Can you work these out from the model? Positions are in its coordinate system, mm. Round coordinates to 2 decimals unless told otherwise and drop trailing zeros. Write each loop counter-clockwise with the first axis right and the second up, starting at its lowest first coordinate (ties: lowest second). Pieces come first, ordered by that corner, then holes. Notation, with made-up numbers: (-31.5, 32) - (16.5, 32) arc R19 ccw to (16.5, 49) - close; hole circle Ø4 at (59, 37.5). An arc over 180 degrees is marked (long way). One line per item, written item: value. Start each with the question number.
(1) If I drill on L1, parallel to X at y = 3.5, z = 0.25; L2, parallel to Z at x = -36, y = 0.25; L3, parallel to X at y = 3.25, z = 1.5, over which ranges is the centre line in solid material (lowest first)? Write a range as from..to.
(2) I want a section at C-C on x = 1.5. List the corners of the cut face in (y, z) for me, plus the area to 3 significant figures.
(3) I want a section at B-B on y = 5.5. Give the number of separate pieces and of enclosed holes in the cut face, plus the area to 3 significant figures.
(4) I want a section at A-A on z = 0. List the corners of the cut face in (x, y) for me, plus the area to 3 significant figures.
(5) I want a section at D-D on x = 36. List the corners of the cut face in (y, z) for me, plus the area to 3 significant figures.
(6) I'm going to push flat-ended pins straight in: pin 1 Ø2 at (x, z) = (-2.5, 3.5) entering from +Y; pin 2 Ø1 at (x, y) = (-9, 1) entering from -Z; pin 3 Ø2 at (x, z) = (13, -2.5) entering from +Y. Where does each tip first touch, or does it pass through?
from build123d import *

# Parameters (mm, degrees)
DODANIE_WYCI_GNI_CIE1_DEPTH                 = 41
DODANIE_WYCI_GNI_CIE1_DEPTH_BACK            = 41
SZKIC2_R                                    = 7.5
WYTNIJ_WYCI_GNI_CIE1_REACH                  = 44.35
WYTNIJ_WYCI_GNI_CIE1_END_RADIUS             = 7.5
SZKIC3_R                                    = 2.5
WYTNIJ_WYCI_GNI_CIE1_DIRECTION_2_REACH      = 44.35
WYTNIJ_WYCI_GNI_CIE1_DIRECTION_2_END_RADIUS = 7.5
SFAZOWANIE1_SIZE                            = 1


with BuildPart() as part:
    # Szkic2 → Dodanie-wyciągnięcie1 (new, two sides: drawn at the far end of the back side and taken through both)
    with BuildSketch(Plane(origin=(0, 0, 0), x_dir=(0, 0, -1), z_dir=(1, 0, 0)).offset(-DODANIE_WYCI_GNI_CIE1_DEPTH_BACK)):
        Circle(SZKIC2_R)
    extrude(amount=DODANIE_WYCI_GNI_CIE1_DEPTH + DODANIE_WYCI_GNI_CIE1_DEPTH_BACK)

    # Wytnij-wyciągnięcie1: up to this cylinder (the profile starts inside it)
    wytnij_wyci_gni_cie1_end = Plane(origin=(0, 0, 0), z_dir=(1, 0, 0)) * Cylinder(WYTNIJ_WYCI_GNI_CIE1_END_RADIUS, 176.7, mode=Mode.PRIVATE)
    # Szkic3 → Wytnij-wyciągnięcie1 (cut, up to the surface)
    with BuildSketch(Plane(origin=(0, 0, 0), x_dir=(1, 0, 0), z_dir=(0, 1, 0)), mode=Mode.PRIVATE) as wytnij_wyci_gni_cie1_sk1:
        with Locations(Location((-36, 0, 0), (0, 0, 90))):
            Circle(SZKIC3_R)
    wytnij_wyci_gni_cie1_tool1 = extrude(wytnij_wyci_gni_cie1_sk1.sketch, amount=-WYTNIJ_WYCI_GNI_CIE1_REACH, mode=Mode.PRIVATE) & wytnij_wyci_gni_cie1_end
    add(wytnij_wyci_gni_cie1_tool1.solids().sort_by_distance((-36, 0, 0))[0], mode=Mode.SUBTRACT)
    # Szkic3 → Wytnij-wyciągnięcie1 (cut, up to the surface)
    with BuildSketch(Plane(origin=(0, 0, 0), x_dir=(1, 0, 0), z_dir=(0, 1, 0)), mode=Mode.PRIVATE) as wytnij_wyci_gni_cie1_sk2:
        with Locations(Location((36, 0, 0), (0, 0, 90))):
            Circle(SZKIC3_R)
    wytnij_wyci_gni_cie1_tool2 = extrude(wytnij_wyci_gni_cie1_sk2.sketch, amount=-WYTNIJ_WYCI_GNI_CIE1_REACH, mode=Mode.PRIVATE) & wytnij_wyci_gni_cie1_end
    add(wytnij_wyci_gni_cie1_tool2.solids().sort_by_distance((36, 0, 0))[0], mode=Mode.SUBTRACT)

    # Wytnij-wyciągnięcie1 direction 2: up to this cylinder (the profile starts inside it)
    wytnij_wyci_gni_cie1_direction_2_end = Plane(origin=(0, 0, 0), z_dir=(1, 0, 0)) * Cylinder(WYTNIJ_WYCI_GNI_CIE1_DIRECTION_2_END_RADIUS, 176.7, mode=Mode.PRIVATE)
    # Szkic3 → Wytnij-wyciągnięcie1 direction 2 (cut, up to the surface)
    with BuildSketch(Plane(origin=(0, 0, 0), x_dir=(1, 0, 0), z_dir=(0, 1, 0)), mode=Mode.PRIVATE) as wytnij_wyci_gni_cie1_direction_2_sk1:
        with Locations(Location((-36, 0, 0), (0, 0, 90))):
            Circle(SZKIC3_R)
    wytnij_wyci_gni_cie1_direction_2_tool1 = extrude(wytnij_wyci_gni_cie1_direction_2_sk1.sketch, amount=WYTNIJ_WYCI_GNI_CIE1_DIRECTION_2_REACH, mode=Mode.PRIVATE) & wytnij_wyci_gni_cie1_direction_2_end
    add(wytnij_wyci_gni_cie1_direction_2_tool1.solids().sort_by_distance((-36, 0, 0))[0], mode=Mode.SUBTRACT)
    # Szkic3 → Wytnij-wyciągnięcie1 direction 2 (cut, up to the surface)
    with BuildSketch(Plane(origin=(0, 0, 0), x_dir=(1, 0, 0), z_dir=(0, 1, 0)), mode=Mode.PRIVATE) as wytnij_wyci_gni_cie1_direction_2_sk2:
        with Locations(Location((36, 0, 0), (0, 0, 90))):
            Circle(SZKIC3_R)
    wytnij_wyci_gni_cie1_direction_2_tool2 = extrude(wytnij_wyci_gni_cie1_direction_2_sk2.sketch, amount=WYTNIJ_WYCI_GNI_CIE1_DIRECTION_2_REACH, mode=Mode.PRIVATE) & wytnij_wyci_gni_cie1_direction_2_end
    add(wytnij_wyci_gni_cie1_direction_2_tool2.solids().sort_by_distance((36, 0, 0))[0], mode=Mode.SUBTRACT)

    # Sfazowanie1
    sfazowanie1_edges = [part.edges().sort_by_distance(p)[0] for p in [
        (-41, 0, 7.5),
        (41, 0, 7.5),
    ]]
    chamfer(sfazowanie1_edges, length=SFAZOWANIE1_SIZE)


solid = part.part
Established:
1. L1: -41..-38.49, -33.51..33.51, 38.49..41
1. L2: -7.5..-2.5, 2.5..7.5
1. L3: -41..-38, -34..34, 38..41
2. outline: circle Ø15 at (0, 0)
2. area: 177 mm2
3. separate pieces: 1
3. enclosed holes: 2
3. area: 794 mm2
4. outline: (-41, -6.5) - (-40, -7.5) - (-38.5, -7.5) - (-38.5, 7.5) - (-40, 7.5) - (-41, 6.5) - close; (-33.5, -7.5) - (33.5, -7.5) - (33.5, 7.5) - (-33.5, 7.5) - close; (38.5, -7.5) - (40, -7.5) - (41, -6.5) - (41, 6.5) - (40, 7.5) - (38.5, 7.5) - close
4. area: 1,080 mm2
5. outline: (-7.07, -2.5) arc R7.5 ccw to (7.07, -2.5) - close; (-7.07, 2.5) - (7.07, 2.5) arc R7.5 ccw to start
5. area: 103 mm2
6. pin 1: y = 7.07
6. pin 2: z = -7.48
6. pin 3: y = 7.35
